from build123d import *

# Parameters (mm, degrees)
BOSS_EXTRUDE1_DEPTH              = 0.5
BOSS_EXTRUDE2_DEPTH              = 5.2
CIRPATTERN1_COUNT                = 4
SKETCH8_R                        = 1.4
BOSS_EXTRUDE4_DEPTH              = 5.9
CIRPATTERN2_COUNT                = 4
FILLET1_R                        = 1
SKETCH11_W                       = 25
SKETCH11_H                       = 25
CUT_EXTRUDE2_DEPTH               = 126.311013881
SKETCH15_R                       = 0.9
CUT_EXTRUDE3_DEPTH               = 126.301756572
SKETCH16_R                       = 1.75
CUT_EXTRUDE4_DEPTH               = 2.3
CBORE_FOR_M1_6_SHCS2_D           = 1.8
CBORE_FOR_M1_6_SHCS2_CBORE_D     = 3.5
CBORE_FOR_M1_6_SHCS2_CBORE_DEPTH = 1.6
SKETCH20_W                       = 0.6
SKETCH20_H                       = 2
CUT_EXTRUDE6_DEPTH               = 5.2
CIRPATTERN3_COUNT                = 4
FILLET2_R                        = 1


with BuildPart() as part:
    # Sketch1 → Boss-Extrude1 (new body)
    with BuildSketch(Plane(origin=(0, 0, 0), x_dir=(1, 0, 0), z_dir=(0, 1, 0))):
        Polygon((0, 0), (0, 6.51), (82, 6.51), (82, 0), (88.51, 0), (88.51, -82), (82, -82), (82, -88.51), (0, -88.51), (0, -82), (-6.51, -82), (-6.51, 0), align=None)
    extrude(amount=BOSS_EXTRUDE1_DEPTH)

    # Sketch2 → Boss-Extrude2 (add)
    with BuildSketch(Plane(origin=(0, 0.5, 0), x_dir=(1, 0, 0), z_dir=(0, 1, 0))):
        with BuildLine():
            Line((41, 6.51), (0, 6.51))
            Line((0, 6.51), (0, 4.51))
            Line((0, 4.51), (39, 4.51))
            Line((39, 4.51), (39, -8.49))
            ThreePointArc((39, -8.49), (51.600076233, -24.910739047), (70.722431864, -16.99))
            Line((70.722431864, -16.99), (74.335460515, -10.732050808))
            Line((74.335460515, -10.732050808), (74.335460515, -6.732050808))
            Line((74.335460515, -6.732050808), (68.990381057, -15.99))
            ThreePointArc((68.990381057, -15.99), (52.117714323, -22.978887394), (41, -8.49))
            Line((41, -8.49), (41, 6.51))
        make_face()
        Polygon((88.51, -41), (88.51, 0), (82, 0), (82, 6.51), (79.094010768, 6.51), (75.335460515, 0), (75.335460515, -4), (86.51, -4), (86.51, -41), align=None)
    boss_extrude2 = extrude(amount=BOSS_EXTRUDE2_DEPTH)

    # CirPattern1: Boss-Extrude2 ×4 about axis
    cirpattern1_axis = Axis((41, 0, 41), (0, 1, 0))
    for i in range(1, CIRPATTERN1_COUNT):
        add(boss_extrude2.rotate(cirpattern1_axis, i * 360 / CIRPATTERN1_COUNT))

    # Sketch8 → Boss-Extrude4 (add)
    with BuildSketch(Plane(origin=(0, 0.5, 0), x_dir=(1, 0, 0), z_dir=(0, 1, 0))):
        with Locations(Location((37, -84.51, 0), (0, 0, 270))):
            Circle(SKETCH8_R)
    boss_extrude4 = extrude(amount=BOSS_EXTRUDE4_DEPTH)

    # CirPattern2: Boss-Extrude4 ×4 about axis
    cirpattern2_axis = Axis((41, 0, 41), (0, 1, 0))
    for i in range(1, CIRPATTERN2_COUNT):
        add(boss_extrude4.rotate(cirpattern2_axis, i * 360 / CIRPATTERN2_COUNT))

    # Fillet1
    fillet1_edges = [part.edges().sort_by_distance(p)[0] for p in [
        (4, 3.1, -4.51),
        (78, 3.1, 86.51),
        (43, 3.1, 86.51),
        (86.51, 3.1, 39),
        (39, 3.1, -4.51),
        (86.51, 3.1, 4),
        (-4.51, 3.1, 78),
        (-4.51, 3.1, 43),
    ]]
    fillet(fillet1_edges, radius=FILLET1_R)

    # Sketch11 → Cut-Extrude2 (cut, through all)
    with BuildSketch(Plane(origin=(0, 0.5, 0), x_dir=(1, 0, 0), z_dir=(0, 1, 0))):
        with Locations((41, -41)):
            Rectangle(SKETCH11_W, SKETCH11_H)
    extrude(amount=-CUT_EXTRUDE2_DEPTH, mode=Mode.SUBTRACT)

    # Sketch15 → Cut-Extrude3 (cut, through all)
    with BuildSketch(Plane(origin=(0, 5.7, 0), x_dir=(1, 0, 0), z_dir=(0, 1, 0))):
        with Locations(Location((81, -78.5, 0), (0, 0, 270))):
            Circle(SKETCH15_R)
        with Locations(Location((78.5, -1, 0), (0, 0, 270))):
            Circle(SKETCH15_R)
        with Locations(Location((1, -3.5, 0), (0, 0, 270))):
            Circle(SKETCH15_R)
        with Locations(Location((3.5, -81, 0), (0, 0, 270))):
            Circle(SKETCH15_R)
    extrude(amount=-CUT_EXTRUDE3_DEPTH, mode=Mode.SUBTRACT)

    # Sketch16 → Cut-Extrude4 (cut)
    with BuildSketch(Plane(origin=(0, 5.7, 0), x_dir=(1, 0, 0), z_dir=(0, 1, 0))):
        with Locations(Location((78.5, -1, 0), (0, 0, 270))):
            Circle(SKETCH16_R)
        with Locations(Location((81, -78.5, 0), (0, 0, 270))):
            Circle(SKETCH16_R)
        with Locations(Location((3.5, -81, 0), (0, 0, 270))):
            Circle(SKETCH16_R)
        with Locations(Location((1, -3.5, 0), (0, 0, 270))):
            Circle(SKETCH16_R)
    extrude(amount=-CUT_EXTRUDE4_DEPTH, mode=Mode.SUBTRACT)

    # CBORE for M1.6 SHCS2 (through all)
    with Locations(Plane(origin=(81, 0, 78.5), x_dir=(0, 0, -1), z_dir=(0, -1, 0))):
        with Locations((0, 0), (77.5, -2.5), (75, -80), (-2.5, -77.5)):
            CounterBoreHole(CBORE_FOR_M1_6_SHCS2_D / 2, CBORE_FOR_M1_6_SHCS2_CBORE_D / 2, CBORE_FOR_M1_6_SHCS2_CBORE_DEPTH)

    # Sketch20 → Cut-Extrude6 (cut)
    with BuildSketch(Plane(origin=(0, 5.7, 0), x_dir=(1, 0, 0), z_dir=(0, 1, 0))):
        with Locations((80.31, -40)):
            Rectangle(SKETCH20_W, SKETCH20_H)
    cut_extrude6 = extrude(amount=-CUT_EXTRUDE6_DEPTH, mode=Mode.SUBTRACT)

    # CirPattern3: Cut-Extrude6 ×4 about axis
    cirpattern3_axis = Axis((41, 0, 41), (0, 1, 0))
    for i in range(1, CIRPATTERN3_COUNT):
        add(cut_extrude6.rotate(cirpattern3_axis, i * 360 / CIRPATTERN3_COUNT), mode=Mode.SUBTRACT)

    # Fillet2
    fillet2_edges = [part.edges().sort_by_distance(p)[0] for p in [
        (0, 2.85, 0),
        (82, 2.85, 0),
        (82, 2.85, 82),
        (0, 2.85, 82),
    ]]
    fillet(fillet2_edges, radius=FILLET2_R)


solid = part.part
Could you check a few things on this model? Use its own coordinates, in mm. A direction names the side the tool comes from. Give positions to 0.01 mm unless a question says otherwise; leave off trailing zeros. Order: outer loops, then holes, each group sorted by start corner. A loop starts at its lowest first (then second) coordinate and runs counter-clockwise, first axis right, second up. Notation, with made-up numbers: (-16, -36.5) - (10, -36.5) arc R11 cw to (10, -24.5) - close; hole circle Ø8 at (-3.5, -32.5). An arc over 180 degrees is marked (long way). One line per item, written item: value. Start each with the question number.
1. For P1, Ø6.5, axis at x = 2.5, z = 63.5, coming from the +Y side; P2, Ø1, axis at x = 69.5, z = 72, coming from the +Y side; P3, Ø2, axis at x = 1, z = 3.5, coming from the -Y side; P4, Ø2.5, axis at y = 3, z = 82.5, coming from the -X side, each with a flat end and sliding along its axis, tell me the tip position at first contact or that it passes through.
2. Thinking about a two-plate mould opening in X: for faces 6 (the face through (43, 3, 83)), 7 (the face through (88.51, 3, 22)), 8 (the face through (5, 3, 41)), which applies, +X half, -X half, draft (parallel to the pull), parting line (faces both ways), or undercut?
3. If I drill on probe 1 along X at (y, z) = (1.75, 81); probe 2 along X at (y, z) = (5.05, 1); probe 3 along X at (y, z) = (5, 56), over which ranges is the centre line in solid material (lowest first)?
4. For faces 1 (the face through (9, 3, 7.665)), 2 (the face through (4, 3.4, 80)), 3 (the face through (-4, 3, 0)), 4 (the face through (4.76, 3.06, 85.3)), 5 (the face through (86, 3, 0)), which set-ups out of +Z, -Z, +X, -X, +Y, -Y let a thin tool reach every point of the face, with its end or its side?
5. Imagine slicing it at A-A on x = 14.5. List the corners of the cut face in (y, z) for me.
Values:
1. P1: y = 0.5
1. P2: y = 5.7
1. P3: y = 1.6
1. P4: x = -6.51
2. face 6: undercut
2. face 7: +X half
2. face 8: draft
3. probe 1: -6.51 to 2.6, 4.4 to 6.66, 41 to 43, 78 to 88.51
3. probe 2: -6.51 to 4, 39 to 41, 75.34 to 76.75, 80.25 to 88.51
3. probe 3: -6.51 to -4.51, 56.51 to 58.51
4. face 1: -X, +Y
4. face 2: +Y
4. face 3: -Z, -X, +Y, -Y
4. face 4: +Z, +Y
4. face 5: -Z, +X, +Y, -Y
5. outline: (0, -6.51) - (5.7, -6.51) - (5.7, -4.51) - (0.5, -4.51) - (0.5, 9.84) - (5.7, 9.84) - (5.7, 12.15) - (0.5, 12.15) - (0.5, 39.74) - (5.7, 39.74) - (5.7, 41.9) - (0.5, 41.9) - (0.5, 60.99) - (5.7, 60.99) - (5.7, 63.88) - (0.5, 63.88) - (0.5, 88.51) - (0, 88.51) - close
